```python
from build123d import *

# Parameters (mm, degrees)
BOSS_EXTRUDE1_DEPTH = 6.35
CUT_EXTRUDE1_DEPTH  = 6.35
FILLET1_R           = 2.54


with BuildPart() as part:
    # Sketch2 → Boss-Extrude1 (new body)
    with BuildSketch(Plane.XY):
        Polygon((-6.35, -63.5), (0, -63.5), (114.3, -38.1), (114.3, 0), (95.377, 0), (95.377, -6.477), (76.073, -6.477), (76.073, 0), (38.227, 0), (38.227, -6.477), (18.923, -6.477), (18.923, 0), (0, 0), (0, -12.7), (-6.35, -12.7), (-6.35, -25.4), (0, -25.4), (0, -50.8), (-6.35, -50.8), align=None)
    extrude(amount=-BOSS_EXTRUDE1_DEPTH)

    # Sketch3 → Cut-Extrude1 (cut)
    with BuildSketch(Plane.XY):
        Polygon((35.837567759, -42.526294431), (9.525, -20.916959432), (9.525, -48.37353171), align=None)
        Polygon((51.284246094, -12.7), (19.530365822, -12.7), (41.715916793, -30.920000703), align=None)
        Polygon((61.141826863, -21.244462208), (51.832146694, -38.971943556), (82.284813735, -32.204684214), align=None)
        Polygon((101.6, -12.7), (72.25424324, -12.7), (101.6, -27.912420599), align=None)
    extrude(amount=-CUT_EXTRUDE1_DEPTH, mode=Mode.SUBTRACT)

    # Fillet1
    fillet1_edges = [part.edges().sort_by_distance(p)[0] for p in [
        (41.715916793, -30.920000703, -3.175),
        (19.530365822, -12.7, -3.175),
        (51.284246094, -12.7, -3.175),
        (61.141826863, -21.244462208, -3.175),
        (82.284813735, -32.204684214, -3.175),
        (51.832146694, -38.971943556, -3.175),
        (72.25424324, -12.7, -3.175),
        (101.6, -12.7, -3.175),
        (101.6, -27.912420599, -3.175),
        (9.525, -20.916959432, -3.175),
        (35.837567759, -42.526294431, -3.175),
        (9.525, -48.37353171, -3.175),
    ]]
    fillet(fillet1_edges, radius=FILLET1_R)


solid = part.part
```
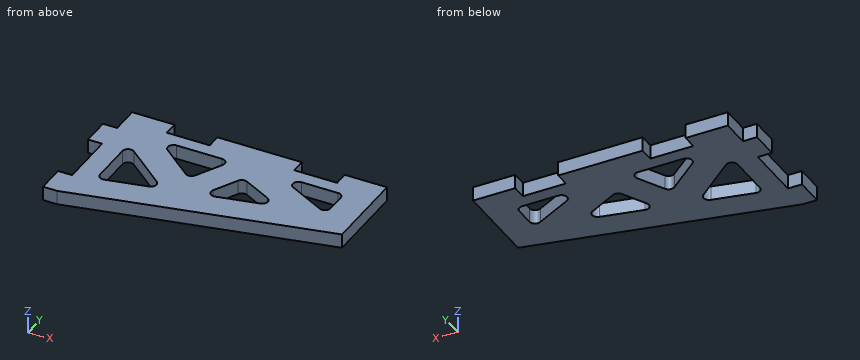
For this review, take the finished solid that the model builds, in its own axes (mm). Coordinates: 2 decimals unless noted, no trailing zeros. Write each loop counter-clockwise with the first axis right and the second up, starting at its lowest first coordinate (ties: lowest second). Pieces come first, ordered by that corner, then holes. Notation, with made-up numbers: (-7.75, 37.5) - (27.25, 37.5) arc R31 ccw to (27.25, 72.5) - close; hole circle Ø11 at (-26.75, 50). An arc over 180 degrees is marked (long way). Answer in a Markdown table with one row per item. Add a question column.
Q1. For probe 1 along X at (y, z) = (-16.5, -3.75); probe 2 along X at (y, z) = (-32, -0.5) (1 decimal); probe 3 along Y at (x, z) = (31, -2.25), list the stretches that pass through material, from the lowest coordinate up.
Q2. We need section A-A, the plane x = 72. State the section outline as (y, z) points.
Q3. For P1, Ø3, axis at x = -2, z = -1.5, coming from the +Y side; P2, Ø3, axis at x = 94.5, z = -3, coming from the -Y side; P3, Ø3, axis at x = 87, z = -4.5, coming from the +Y side, all flat-tipped, find the tip position at first contact; note any pin that passes through.
Q4. We need section B-B, the plane z = -4. Count the separate pieces of the cut face and the enclosed holes in it, and give its area (3 significant figures).
Q5. We need section D-D, the plane y = -56. State the section outline as (x, z) points, and give its area (3 significant figures).
Q6. We need section C-C, the plane x = 41. State the section outline as (y, z) points.
Answer list:
| question | item | result |
|---|---|---|
| 1 | probe 1 | x = -6.35 to 24.42, 49.29 to 80.47, 101.6 to 114.3 |
| 1 | probe 2 | x = 0 to 9.5, 23 to 55.5, 77.3 to 114.3 |
| 1 | probe 3 | y = -56.61 to -43.59, -38.55 to -22.12, -12.7 to -6.48 |
| 2 | outline | (-47.5, -6.35) - (-34.49, -6.35) - (-34.49, 0) - (-47.5, 0) - close; (-26.87, -6.35) - (0, -6.35) - (0, 0) - (-26.87, 0) - close |
| 3 | P1 | stops at y = -12.7 |
| 3 | P2 | stops at y = -42.83 |
| 3 | P3 | stops at y = -6.48 |
| 4 | separate pieces | 1 |
| 4 | enclosed holes | 4 |
| 4 | area | 4,680 mm2 |
| 5 | outline | (-6.35, -6.35) - (33.75, -6.35) - (33.75, 0) - (-6.35, 0) - close |
| 5 | area | 255 mm2 |
| 6 | outline | (-54.39, -6.35) - (-29.52, -6.35) - (-29.52, 0) - (-54.39, 0) - close; (-12.7, -6.35) - (0, -6.35) - (0, 0) - (-12.7, 0) - close |
